Design review of the part built by this model. Coordinates are the model's own, in mm. A direction names the side the tool comes from. Round coordinates to 2 decimals unless told otherwise and drop trailing zeros. Write each loop counter-clockwise with the first axis right and the second up, starting at its lowest first coordinate (ties: lowest second). Pieces come first, ordered by that corner, then holes. Notation, with made-up numbers: M 76.25,28 L 135.25,28 A20 ccw 135.25,65 Z; hole C 66,-26.75 d8. An arc over 180 degrees is marked long. One line per question, with ' | ' between items. Start each with the question number.
Item 1: Draft analysis for pull direction X (two halves, no side actions). For faces 6 (the face through (-34.36, -4.93, -20.16)), 7 (the face through (12, 0, 1)), 8 (the face through (-8.926, -1.479, -38.334)), 9 (the face through (-41.804, -4.93, 24.588)), state which applies: released by +X, released by -X, zero draft, split by the parting line, or undercut.
Item 2: Add section B-B, the plane z = 5. State the section outline as (x, y) points, and give its area (3 significant figures).
Item 3: Machinability: for faces 1 (the face through (0, -5, 48.497)), 2 (the face through (32.025, -4.837, 29.736)), 3 (the face through (-7.51, -4.24, -42.6)), 4 (the face through (45.226, -4.93, 0.037)), 5 (the face through (0, -6, -39.837)), which of the approach directions +Z, -Z, +X, -X, +Y, -Y give a long, thin tool a straight path to every point of the face, cutting with its end or side? Answer none if there is none.
Item 4: For L1, parallel to Y at x = 8.5, z = 41.45; L2, parallel to X at y = -2, z = -20.5; L3, parallel to X at y = -6.5, z = -28.5, list the stretches that pass through material, from the lowest coordinate up.
Item 5: Insertion check: pin 1 Ø5.5 at (x, y) = (8.5, -5) entering from +Z; pin 2 Ø4 at (x, y) = (-8.5, -5) entering from +Z; pin 3 Ø1 at (y, z) = (-8, 3.5) entering from +X. Each pin has a flat end and moves straight along its axis. Give the tip position at first contact, or say it passes through.
Item 6: Add section A-A, the plane x = 0. State the section outline as (y, z) points, and give its area (3 significant figures).
Item 7: Add section C-C, the plane y = -5. Give the number of separate pieces and of enclosed holes in the cut face, and give its area (3 significant figures).
```python
from build123d import *

# Parameters (mm, degrees)
F0_R      = 9.0451569713
F1_DEPTH  = 3
F2_DEPTH  = 10
F8_D      = 6
F8_DEPTH  = 2
F8_TIP    = 1.8025818571
F9_D      = 2.5
F9_DEPTH  = 13.5
F9_START  = 3.0515061
F9_TIP    = 0.7510757738
F10_D     = 2.5
F10_DEPTH = 13.5
F10_TIP   = 0.7510757738
F11_D     = 6
F11_DEPTH = 2
F11_TIP   = 1.8025818571
F12_D     = 6
F12_DEPTH = 2
F12_TIP   = 1.8025818571
F13_D     = 2.5
F13_DEPTH = 13.5
F13_START = 3.0515061
F13_TIP   = 0.7510757738
F15_D     = 2.5
F15_DEPTH = 13.5
F15_TIP   = 0.7510757738
F16_D     = 6
F16_DEPTH = 2
F16_TIP   = 1.8025818571
F17_D     = 6
F17_DEPTH = 2
F17_TIP   = 1.8025818571
F18_D     = 2.5
F18_DEPTH = 13.5
F18_START = 3.0515061
F18_TIP   = 0.7510757738
F19_D     = 2.5
F19_DEPTH = 13.5
F19_TIP   = 0.7510757738
F20_D     = 6
F20_DEPTH = 2
F20_TIP   = 1.8025818571
F21_D     = 5.1054
F21_DEPTH = 15.81
F21_TIP   = 1.5338169022


with BuildPart() as f1:
    # F0 (on Front) → F1 (new body)
    with BuildSketch(Plane.XZ):
        Polygon((28, -48.4974226119), (56, 0), (28, 48.4974226119), (-28, 48.4974226119), (-56, 0), (-28, -48.4974226119), align=None)
        with BuildLine():
            ThreePointArc((44.556624327, 2.5), (45.2264973081, 0), (44.556624327, -2.5))
            Line((44.556624327, -2.5), (24.443375673, -37.3371685741))
            ThreePointArc((24.443375673, -37.3371685741), (22.6132486541, -39.167295593), (20.1132486541, -39.8371685741))
            Line((20.1132486541, -39.8371685741), (12.5, -39.8371685741))
            Line((12.5, -39.8371685741), (-12.5, -39.8371685741))
            Line((-12.5, -39.8371685741), (-20.1132486541, -39.8371685741))
            ThreePointArc((-20.1132486541, -39.8371685741), (-22.6132486541, -39.167295593), (-24.443375673, -37.3371685741))
            Line((-24.443375673, -37.3371685741), (-44.556624327, -2.5))
            ThreePointArc((-44.556624327, -2.5), (-45.2264973081, 0), (-44.556624327, 2.5))
            Line((-44.556624327, 2.5), (-40.75, 9.0932667397))
            Line((-40.75, 9.0932667397), (-28.25, 30.7439018343))
            Line((-28.25, 30.7439018343), (-24.443375673, 37.3371685741))
            ThreePointArc((-24.443375673, 37.3371685741), (-22.6132486541, 39.167295593), (-20.1132486541, 39.8371685741))
            Line((-20.1132486541, 39.8371685741), (20.1132486541, 39.8371685741))
            ThreePointArc((20.1132486541, 39.8371685741), (22.6132486541, 39.167295593), (24.443375673, 37.3371685741))
            Line((24.443375673, 37.3371685741), (28.25, 30.7439018343))
            Line((28.25, 30.7439018343), (40.75, 9.0932667397))
            Line((40.75, 9.0932667397), (44.556624327, 2.5))
        make_face(mode=Mode.SUBTRACT)
        with BuildLine():
            ThreePointArc((33.9198729811, 10.9233937587), (37.7139682066, 11.4228958712), (40.75, 9.0932667397))
            Line((40.75, 9.0932667397), (28.25, 30.7439018343))
            ThreePointArc((28.25, 30.7439018343), (28.7495021125, 26.9498066088), (26.4198729811, 23.9137748154))
            Line((26.4198729811, 23.9137748154), (2.5, 10.1036297108))
            ThreePointArc((2.5, 10.1036297108), (0, 9.4337567297), (-2.5, 10.1036297108))
            Line((-2.5, 10.1036297108), (-26.4198729811, 23.9137748154))
            ThreePointArc((-26.4198729811, 23.9137748154), (-28.7495021125, 26.9498066088), (-28.25, 30.7439018343))
            Line((-28.25, 30.7439018343), (-40.75, 9.0932667397))
            ThreePointArc((-40.75, 9.0932667397), (-37.7139682066, 11.4228958712), (-33.9198729811, 10.9233937587))
            Line((-33.9198729811, 10.9233937587), (-10, -2.8867513459))
            ThreePointArc((-10, -2.8867513459), (-8.1698729811, -4.7168783649), (-7.5, -7.2168783649))
            Line((-7.5, -7.2168783649), (-7.5, -34.8371685741))
            ThreePointArc((-7.5, -34.8371685741), (-8.9644660941, -38.37270248), (-12.5, -39.8371685741))
            Line((-12.5, -39.8371685741), (12.5, -39.8371685741))
            ThreePointArc((12.5, -39.8371685741), (8.9644660941, -38.37270248), (7.5, -34.8371685741))
            Line((7.5, -34.8371685741), (7.5, -7.2168783649))
            ThreePointArc((7.5, -7.2168783649), (8.1698729811, -4.7168783649), (10, -2.8867513459))
            Line((10, -2.8867513459), (33.9198729811, 10.9233937587))
        make_face()
        Circle(F0_R, mode=Mode.SUBTRACT)
        Circle(F0_R)
    extrude(amount=F1_DEPTH)

    # F0 (on Front) → F2 (join)
    with BuildSketch(Plane.XZ):
        Polygon((28, -48.4974226119), (56, 0), (28, 48.4974226119), (-28, 48.4974226119), (-56, 0), (-28, -48.4974226119), align=None)
        with BuildLine():
            ThreePointArc((44.556624327, 2.5), (45.2264973081, 0), (44.556624327, -2.5))
            Line((44.556624327, -2.5), (24.443375673, -37.3371685741))
            ThreePointArc((24.443375673, -37.3371685741), (22.6132486541, -39.167295593), (20.1132486541, -39.8371685741))
            Line((20.1132486541, -39.8371685741), (12.5, -39.8371685741))
            Line((12.5, -39.8371685741), (-12.5, -39.8371685741))
            Line((-12.5, -39.8371685741), (-20.1132486541, -39.8371685741))
            ThreePointArc((-20.1132486541, -39.8371685741), (-22.6132486541, -39.167295593), (-24.443375673, -37.3371685741))
            Line((-24.443375673, -37.3371685741), (-44.556624327, -2.5))
            ThreePointArc((-44.556624327, -2.5), (-45.2264973081, 0), (-44.556624327, 2.5))
            Line((-44.556624327, 2.5), (-40.75, 9.0932667397))
            Line((-40.75, 9.0932667397), (-28.25, 30.7439018343))
            Line((-28.25, 30.7439018343), (-24.443375673, 37.3371685741))
            ThreePointArc((-24.443375673, 37.3371685741), (-22.6132486541, 39.167295593), (-20.1132486541, 39.8371685741))
            Line((-20.1132486541, 39.8371685741), (20.1132486541, 39.8371685741))
            ThreePointArc((20.1132486541, 39.8371685741), (22.6132486541, 39.167295593), (24.443375673, 37.3371685741))
            Line((24.443375673, 37.3371685741), (28.25, 30.7439018343))
            Line((28.25, 30.7439018343), (40.75, 9.0932667397))
            Line((40.75, 9.0932667397), (44.556624327, 2.5))
        make_face(mode=Mode.SUBTRACT)
        Circle(F0_R)
    extrude(amount=F2_DEPTH)

    # F8
    with Locations(Plane(origin=(0, 0, -48.4974226119), x_dir=(1, 0, 0), z_dir=(0, 0, -1))):
        with Locations((-8.5, 5), (8.5, 5)):
            Hole(F8_D / 2, depth=F8_DEPTH)
            with Locations((0, 0, -(F8_DEPTH + F8_TIP / 2))):  # 118° drill point
                Cone(0, F8_D / 2, F8_TIP, mode=Mode.SUBTRACT)

    # F9
    # its depths count from where the whole tool has entered the part; down to there all is cleared
    with Locations(Plane(origin=(0, 0, -48.4974226119), x_dir=(1, 0, 0), z_dir=(0, 0, -1)).offset(-F9_START)):
        with Locations((-8.5, 5), (8.5, 5)):
            Hole(F9_D / 2, depth=F9_DEPTH)
            with Locations((0, 0, -(F9_DEPTH + F9_TIP / 2))):  # 118° drill point
                Cone(0, F9_D / 2, F9_TIP, mode=Mode.SUBTRACT)

    # F10
    with Locations(Plane(origin=(42, 0, -24.248711306), x_dir=(0, 1, 0), z_dir=(0.8660254038, 0, -0.5))):
        with Locations((-5, -8.5), (-5, 8.5)):
            Hole(F10_D / 2, depth=F10_DEPTH)
            with Locations((0, 0, -(F10_DEPTH + F10_TIP / 2))):  # 118° drill point
                Cone(0, F10_D / 2, F10_TIP, mode=Mode.SUBTRACT)

    # F11
    with Locations(Plane(origin=(42, 0, -24.248711306), x_dir=(0, 1, 0), z_dir=(0.8660254038, 0, -0.5))):
        with Locations((-5, -8.5), (-5, 8.5)):
            Hole(F11_D / 2, depth=F11_DEPTH)
            with Locations((0, 0, -(F11_DEPTH + F11_TIP / 2))):  # 118° drill point
                Cone(0, F11_D / 2, F11_TIP, mode=Mode.SUBTRACT)

    # F12
    with Locations(Plane(origin=(42, 0, 24.248711306), x_dir=(0, 1, 0), z_dir=(0.8660254038, 0, 0.5))):
        with Locations((-5, -8.5), (-5, 8.5)):
            Hole(F12_D / 2, depth=F12_DEPTH)
            with Locations((0, 0, -(F12_DEPTH + F12_TIP / 2))):  # 118° drill point
                Cone(0, F12_D / 2, F12_TIP, mode=Mode.SUBTRACT)

    # F13
    # its depths count from where the whole tool has entered the part; down to there all is cleared
    with Locations(Plane(origin=(42, 0, 24.248711306), x_dir=(0, 1, 0), z_dir=(0.8660254038, 0, 0.5)).offset(-F13_START)):
        with Locations((-5, -8.5), (-5, 8.5)):
            Hole(F13_D / 2, depth=F13_DEPTH)
            with Locations((0, 0, -(F13_DEPTH + F13_TIP / 2))):  # 118° drill point
                Cone(0, F13_D / 2, F13_TIP, mode=Mode.SUBTRACT)

    # F15
    with Locations(Plane.XY.offset(48.4974226119)):
        with Locations((8.5, -5), (-8.5, -5)):
            Hole(F15_D / 2, depth=F15_DEPTH)
            with Locations((0, 0, -(F15_DEPTH + F15_TIP / 2))):  # 118° drill point
                Cone(0, F15_D / 2, F15_TIP, mode=Mode.SUBTRACT)

    # F16
    with Locations(Plane.XY.offset(48.4974226119)):
        with Locations((8.5, -5), (-8.5, -5)):
            Hole(F16_D / 2, depth=F16_DEPTH)
            with Locations((0, 0, -(F16_DEPTH + F16_TIP / 2))):  # 118° drill point
                Cone(0, F16_D / 2, F16_TIP, mode=Mode.SUBTRACT)

    # F17
    with Locations(Plane(origin=(-42, 0, 24.248711306), x_dir=(0, -1, 0), z_dir=(-0.8660254038, 0, 0.5))):
        with Locations((5, 8.5), (5, -8.5)):
            Hole(F17_D / 2, depth=F17_DEPTH)
            with Locations((0, 0, -(F17_DEPTH + F17_TIP / 2))):  # 118° drill point
                Cone(0, F17_D / 2, F17_TIP, mode=Mode.SUBTRACT)

    # F18
    # its depths count from where the whole tool has entered the part; down to there all is cleared
    with Locations(Plane(origin=(-42, 0, 24.248711306), x_dir=(0, -1, 0), z_dir=(-0.8660254038, 0, 0.5)).offset(-F18_START)):
        with Locations((5, 8.5), (5, -8.5)):
            Hole(F18_D / 2, depth=F18_DEPTH)
            with Locations((0, 0, -(F18_DEPTH + F18_TIP / 2))):  # 118° drill point
                Cone(0, F18_D / 2, F18_TIP, mode=Mode.SUBTRACT)

    # F19
    with Locations(Plane(origin=(-42, 0, -24.248711306), x_dir=(0, -1, 0), z_dir=(-0.8660254038, 0, -0.5))):
        with Locations((5, 8.5), (5, -8.5)):
            Hole(F19_D / 2, depth=F19_DEPTH)
            with Locations((0, 0, -(F19_DEPTH + F19_TIP / 2))):  # 118° drill point
                Cone(0, F19_D / 2, F19_TIP, mode=Mode.SUBTRACT)

    # F20
    with Locations(Plane(origin=(-42, 0, -24.248711306), x_dir=(0, -1, 0), z_dir=(-0.8660254038, 0, -0.5))):
        with Locations((5, 8.5), (5, -8.5)):
            Hole(F20_D / 2, depth=F20_DEPTH)
            with Locations((0, 0, -(F20_DEPTH + F20_TIP / 2))):  # 118° drill point
                Cone(0, F20_D / 2, F20_TIP, mode=Mode.SUBTRACT)

    # F21
    with Locations(Plane(origin=(0, 0, 0), x_dir=(1, 0, 0), z_dir=(0, 1, 0))):
        with Locations((0, 0)):
            Hole(F21_D / 2, depth=F21_DEPTH)
            with Locations((0, 0, -(F21_DEPTH + F21_TIP / 2))):  # 118° drill point
                Cone(0, F21_D / 2, F21_TIP, mode=Mode.SUBTRACT)


solid = f1.part
```
Computed values:
1) face 6: undercut | face 7: zero draft | face 8: undercut | face 9: released by -X
2) outline: M -53.11,-10 L -43.11,-10 L -43.11,0 L -53.11,0 Z; M -23.66,-3 L -7.54,-3 L -7.54,-10 L 7.54,-10 L 7.54,-3 L 23.66,-3 L 23.66,0 L -23.66,0 Z; M 43.11,-10 L 53.11,-10 L 53.11,0 L 43.11,0 Z | area: 447 mm^2
3) face 1: +Z, +X, -X, +Y, -Y | face 2: none | face 3: -Z | face 4: +Y, -Y | face 5: -Y
4) L1: y = -10 to -6.25, -3.75 to 0 | L2: x = -44.16 to -34.16, -7.5 to 7.5, 34.16 to 44.16 | L3: x = -39.55 to -37.56, -37.1 to -29.55, 29.55 to 37.1, 37.56 to 39.55
5) pin 1: stops at z = 46.35 | pin 2: stops at z = 45.9 | pin 3: stops at x = 54.27
6) outline: M -10,-48.5 L 0,-48.5 L 0,-2.55 L -10,-2.55 L -10,-9.05 L -3,-9.05 L -3,-39.84 L -10,-39.84 Z; M -10,2.55 L 0,2.55 L 0,9.43 L -3,9.43 L -3,9.05 L -10,9.05 Z; M -10,39.84 L 0,39.84 L 0,48.5 L -10,48.5 Z | area: 397 mm^2
7) separate pieces: 13 | enclosed holes: 1 | area: 2,530 mm^2
